Can you work these out from the model? Positions are in its coordinate system, mm. A direction names the side the tool comes from. Give positions to 0.01 mm unless a question says otherwise; leave off trailing zeros. Write each loop counter-clockwise with the first axis right and the second up, starting at its lowest first coordinate (ties: lowest second). Pieces come first, ordered by that corner, then holes.
from build123d import *

# Parameters (mm, degrees)
F1_DEPTH = 1.5


with BuildPart() as f1:
    # F0 (on Top) → F1 (new body)
    with BuildSketch(Plane.XY):
        with BuildLine():
            ThreePointArc((0, 3), (0.87868, 0.87868), (3, 0))
            Line((3, 0), (7, 0))
            ThreePointArc((7, 0), (9.12132, 0.87868), (10, 3))
            ThreePointArc((10, 3), (9.12132, 5.12132), (7, 6))
            Line((7, 6), (5, 6))
            Line((5, 6), (5, 5.2))
            Line((5, 5.2), (7, 5.2))
            ThreePointArc((7, 5.2), (8.555635, 4.555635), (9.2, 3))
            ThreePointArc((9.2, 3), (8.555635, 1.444365), (7, 0.8))
            Line((7, 0.8), (3, 0.8))
            ThreePointArc((3, 0.8), (1.444365, 1.444365), (0.8, 3))
            ThreePointArc((0.8, 3), (1.444365, 4.555635), (3, 5.2))
            Line((3, 5.2), (4, 5.2))
            Line((4, 5.2), (4, 6))
            Line((4, 6), (3, 6))
            ThreePointArc((3, 6), (0.87868, 5.12132), (0, 3))
        make_face()
    extrude(amount=F1_DEPTH)


solid = f1.part
(1) For faces 3 (the face through (5, 0.8, 1)), 4 (the face through (6, 6, 1)), which set-ups out of +Z, -Z, +X, -X, +Y, -Y let a thin tool reach every point of the face, with its end or its side?
Returned:
face 3: +Z, -Z
face 4: +Z, -Z, +X, -X, +Y
(2) If I drill on L1, parallel to X at y = 3, z = 1.15; L2, parallel to Y at x = 7, z = 0.8; L3, parallel to X at y = 2.25, z = 1.3, over which ranges is the centre line in solid material (lowest first)?
Returned:
L1: x = 0 to 0.8, 9.2 to 10
L2: y = 0 to 0.8, 5.2 to 6
L3: x = 0.1 to 0.93, 9.07 to 9.9
(3) Imagine slicing it at B-B, the plane z = 0.95. Write out the boundary of the cut face in (x, y).
Returned:
outline: (0, 3) arc R3 ccw to (3, 0) - (7, 0) arc R3 ccw to (10, 3) arc R3 ccw to (7, 6) - (5, 6) - (5, 5.2) - (7, 5.2) arc R2.2 cw to (7, 0.8) - (3, 0.8) arc R2.2 cw to (3, 5.2) - (4, 5.2) - (4, 6) - (3, 6) arc R3 ccw to start
(4) If we mould it in two halves opening along X, with no side actions, what happens to faces 1 (the face through (5, 0.6, 1.5)), 2 (the face through (6, 5.2, 1))? For each: +X half, -X half, draft (parallel to the pull), parting line (faces both ways), or undercut.
Returned:
face 1: draft
face 2: undercut
(5) Imagine slicing it at A-A, the plane y = 2.25. Write out the boundary of the cut face in (x, z).
Returned:
outline: (0.1, 0) - (0.93, 0) - (0.93, 1.5) - (0.1, 1.5) - close; (9.07, 0) - (9.9, 0) - (9.9, 1.5) - (9.07, 1.5) - close
(6) Will this pin go through, and if not, where does the flat tip stop? P1, Ø0.6, axis at y = 5.5, z = 1, coming from the +X side.
Returned:
P1: stops at x = 9.04
(7) Imagine slicing it at C-C, the plane x = 8.5. Write out the boundary of the cut face in (y, z).
Returned:
outline: (0.4, 0) - (1.39, 0) - (1.39, 1.5) - (0.4, 1.5) - close; (4.61, 0) - (5.6, 0) - (5.6, 1.5) - (4.61, 1.5) - close
(8) Imagine slicing it at D-D, the plane x = 4.75. Write out the boundary of the cut face in (y, z), plus the area to 3 significant figures.
Returned:
outline: (0, 0) - (0.8, 0) - (0.8, 1.5) - (0, 1.5) - close
area: 1.20 mm2
